```python
from build123d import *

# Parameters (mm, degrees)
SKETCH1_W           = 30
SKETCH1_H           = 3.002768409
SKETCH1_H_2         = 3
BOSS_EXTRUDE1_DEPTH = 3


with BuildPart() as part:
    # Sketch1 → Boss-Extrude1 (new body)
    with BuildSketch(Plane(origin=(0, 0, 0), x_dir=(1, 0, 0), z_dir=(0, 1, 0))):
        Polygon((0, 31), (0, 42), (302, 42), (302, 31), (299, 31), (299, 11), (302, 11), (302, 0), (0, 0), (0, 11), (3, 11), (3, 31), align=None)
        with Locations((244, 4.501384205)):
            Rectangle(SKETCH1_W, SKETCH1_H, mode=Mode.SUBTRACT)
        with Locations((58, 37.497231591)):
            Rectangle(SKETCH1_W, SKETCH1_H_2, mode=Mode.SUBTRACT)
        with Locations((151, 37.5)):
            Rectangle(SKETCH1_W, SKETCH1_H_2, mode=Mode.SUBTRACT)
        with Locations((244, 37.498615796)):
            Rectangle(SKETCH1_W, SKETCH1_H, mode=Mode.SUBTRACT)
        with Locations((151, 4.5)):
            Rectangle(SKETCH1_W, SKETCH1_H_2, mode=Mode.SUBTRACT)
        with Locations((58, 4.502768409)):
            Rectangle(SKETCH1_W, SKETCH1_H_2, mode=Mode.SUBTRACT)
    extrude(amount=BOSS_EXTRUDE1_DEPTH)


solid = part.part
```
Geometry: final body of the model. Coordinates: model frame, mm. Round coordinates to 2 decimals unless told otherwise and drop trailing zeros. Write each loop counter-clockwise with the first axis right and the second up, starting at its lowest first coordinate (ties: lowest second). Pieces come first, ordered by that corner, then holes. Notation, with made-up numbers: (-15.75, 4) -> (26.25, 4) arc R11 cw to (26.25, 11) -> close; hole circle Ø4 at (9.5, -38.5). An arc over 180 degrees is marked (long way). Return JSON: item names as keys, results as strings.
Q1. First-contact query: pin 1 Ø1 at (y, z) = (1, -27) entering from +X. Flat tip, straight axial feed; report the tip coordinate or a pass-through.
From the geometry:
{"pin 1": "x = 299"}
Q2. Section A-A on z = -16.5. Return the cut outline in (x, y).
From the geometry:
{"outline": "(3, 0) -> (299, 0) -> (299, 3) -> (3, 3) -> close"}
Q3. Section B-B on y = 1.75. Give the number of separate pieces and of enclosed holes in the cut face, and give its area (3 significant figures).
From the geometry:
{"separate pieces": "1", "enclosed holes": "6", "area": "12,000 mm2"}
Q4. Ray query, line 1 (Z direction, x = 145, y = 0.85); line 2 (X direction, y = 2.75, z = -5); line 3 (X direction, y = 2.1, z = -16). Return the intervals inside material, ascending.
From the geometry:
{"line 1": "-42 to -39, -36 to -6, -3 to 0", "line 2": "0 to 43, 73 to 136, 166 to 229, 259 to 302", "line 3": "3 to 299"}
